The drawing under review shows one solid part. Ordinate dimensions are in mm from its lowest x, y, z. Give positions to 0.01 mm unless a question says otherwise; leave off trailing zeros. Order: outer loops, then holes, each group sorted by start corner. A loop starts at its lowest first (then second) coordinate and runs counter-clockwise, first axis right, second up. Notation, with made-up numbers: (22.5, 75) -> (54.5, 75) arc R17 cw to (54.5, 104) -> close; hole circle Ø1 at (-16.5, 55). An arc over 180 degrees is marked (long way). Return JSON: item names as keys, results as strings. Group by question number.
1) Add section A-A (z = 154). Give the boundary of the cut face in (x, y), then the cut area to 3 significant figures.
2) To check wall thickness, follow line 1 along X through (y, z) = (25.5, 158.5) (1 decimal); line 2 along X through (y, z) = (26.75, 123) (1 decimal); line 3 along Z through (x, y) = (46, 20.75). State the ranges of each line that lie inside material, in increasing order.
3) Add section D-D (z = 17). Give the boundary of the cut face in (x, y).
4) The part is to be moulded in two halves that separate along Z. For the marked faces 1 and 2, say which applies: released by +Z, released by -Z, zero draft, split by the parting line, or undercut.
5) Add section C-C (x = 162.5). Give the boundary of the cut face in (y, z).
6) Add section B-B (y = 7). Give the boundary of the cut face in (x, z) (1 decimal).
7) Insertion check: P1, Ø4.5, axis at y = 22, z = 4.5, coming from the -X side; P2, Ø2.5, axis at x = 146.5, y = 12, coming from the +Z side; P3, Ø2.5, axis at x = 146, y = 18, coming from the -Z side; P4, Ø2, axis at y = 5.5, z = 44.5, coming from the -X side. Each pin has a flat end and moves straight along its axis. Give the tip position at first contact, or say it passes through.
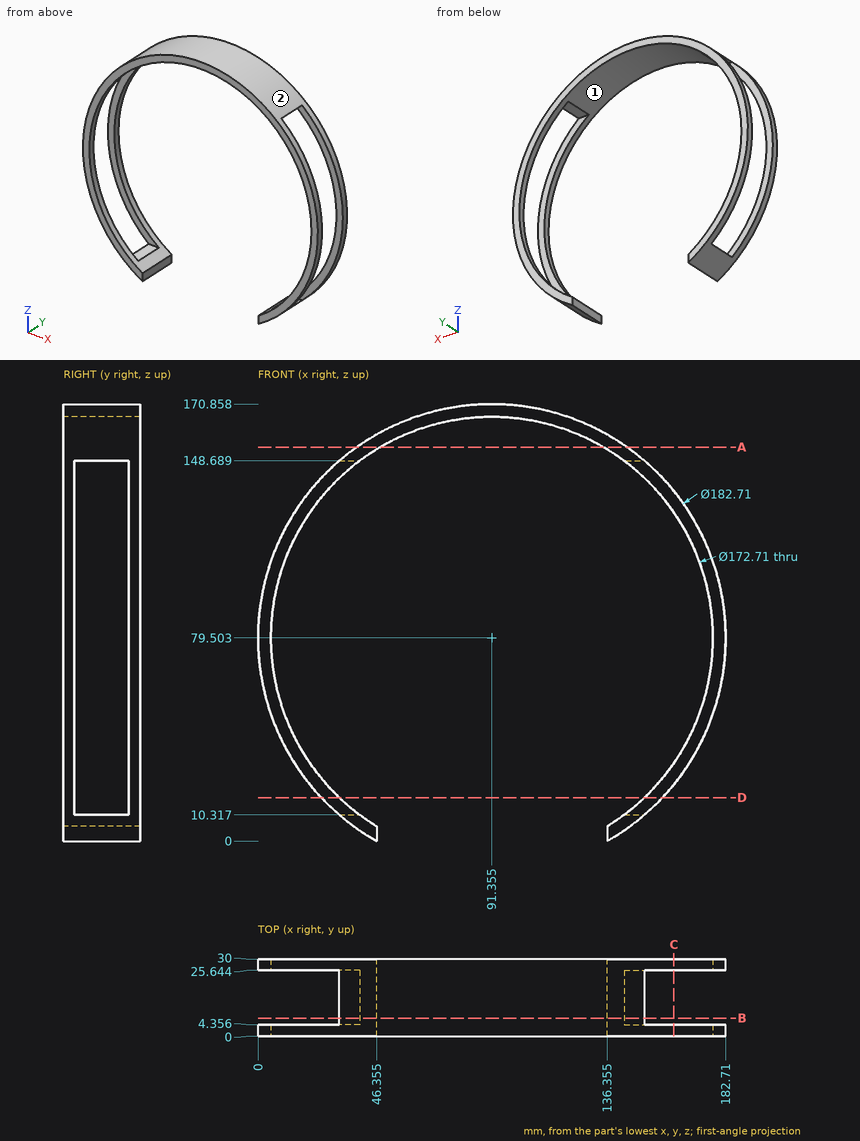
Evaluation:
{
 "1": {"outline": "(38.48, 0) -> (47.68, 0) -> (47.68, 30) -> (38.48, 30) -> close; (135.03, 0) -> (144.23, 0) -> (144.23, 30) -> (135.03, 30) -> close", "area": "552 mm^2"},
 "2": {"line 1": "45.5 to 56.5, 126.2 to 137.2", "line 2": "11 to 16.8, 166 to 171.7", "line 3": "0.2 to 6.02, 152.99 to 158.8"},
 "3": {"outline": "(24.73, 0) -> (31.77, 0) -> (31.77, 4.36) -> (24.73, 4.36) -> close; (24.73, 25.64) -> (31.77, 25.64) -> (31.77, 30) -> (24.73, 30) -> close; (150.94, 0) -> (157.98, 0) -> (157.98, 4.36) -> (150.94, 4.36) -> close; (150.94, 25.64) -> (157.98, 25.64) -> (157.98, 30) -> (150.94, 30) -> close"},
 "4": {"face 1": "undercut", "face 2": "split by the parting line"},
 "5": {"outline": "(0, 22.2) -> (4.36, 22.2) -> (4.36, 30.56) -> (0, 30.56) -> close; (0, 128.45) -> (4.36, 128.45) -> (4.36, 136.81) -> (0, 136.81) -> close; (25.64, 22.2) -> (30, 22.2) -> (30, 30.56) -> (25.64, 30.56) -> close; (25.64, 128.45) -> (30, 128.45) -> (30, 136.81) -> (25.64, 136.81) -> close"},
 "6": {"outline": "(31.7, 10.3) arc R91.4 ccw to (46.4, 0) -> (46.4, 5.8) arc R86.4 cw to (39.7, 10.3) -> close; (31.7, 148.7) -> (39.7, 148.7) arc R86.4 cw to (143, 148.7) -> (151, 148.7) arc R91.4 ccw to start; (136.4, 0) arc R91.4 ccw to (151, 10.3) -> (143, 10.3) arc R86.4 cw to (136.4, 5.8) -> close"},
 "7": {"P1": "x = 36.1", "P2": "z = 153.27", "P3": "z = 5.38", "P4": "through"}
}
